The figure shows three views and two pictorial views of one solid part (mm, origin at its lowest corner). Answer the questions. Coordinates: 2 decimals unless noted, no trailing zeros. Loops run counter-clockwise (first coordinate to the right, second up) from the corner with the lowest first, then second, coordinate; pieces in that order, holes last. Notation, with made-up numbers: M 46.5,-7 L 104.5,-7 A22 ccw 104.5,25 Z; hole C -32.5,21 d9. An arc over 180 degrees is marked long. Return JSON: item names as keys, results as strings. Group by question number.
1. Section C-C (x = 32.25) is taken. Write down the section's boundary in (y, z).
2. Section D-D (z = 30) is taken. Write down the section's boundary in (x, y), then the cut area to 3 significant figures.
3. Given P1, Ø6, axis at x = 36.5, y = 23, coming from the -Z side; P2, Ø1, axis at x = 69.5, z = 93.5, coming from the +Y side; P3, Ø4, axis at y = 28.5, z = 33.5, coming from the -X side, each flat-ended and moving along its own axis, determine where each tip first touches the part or whether it passes through.
4. The mould has two halves that part along X. Classify the marked faces 1 and 2: pulls with the +X half, pulls with the -X half, needs draft (parallel to the pull), parting line crosses it, or undercut.
5. Section B-B (y = 32) is taken. Write down the section's boundary in (x, z), then the cut area to 3 significant figures.
6. Straight lines are drawn through the part: L1, parallel to Y at x = 89, z = 95; L2, parallel to X at y = 29, z = 33.5; L3, parallel to X at y = 19.5, z = 28. For each, find the intervals that lie inside material, in ascending order. Write a range as from..to.
7. Section A-A (z = 90) is taken. Write down the section's boundary in (x, y).
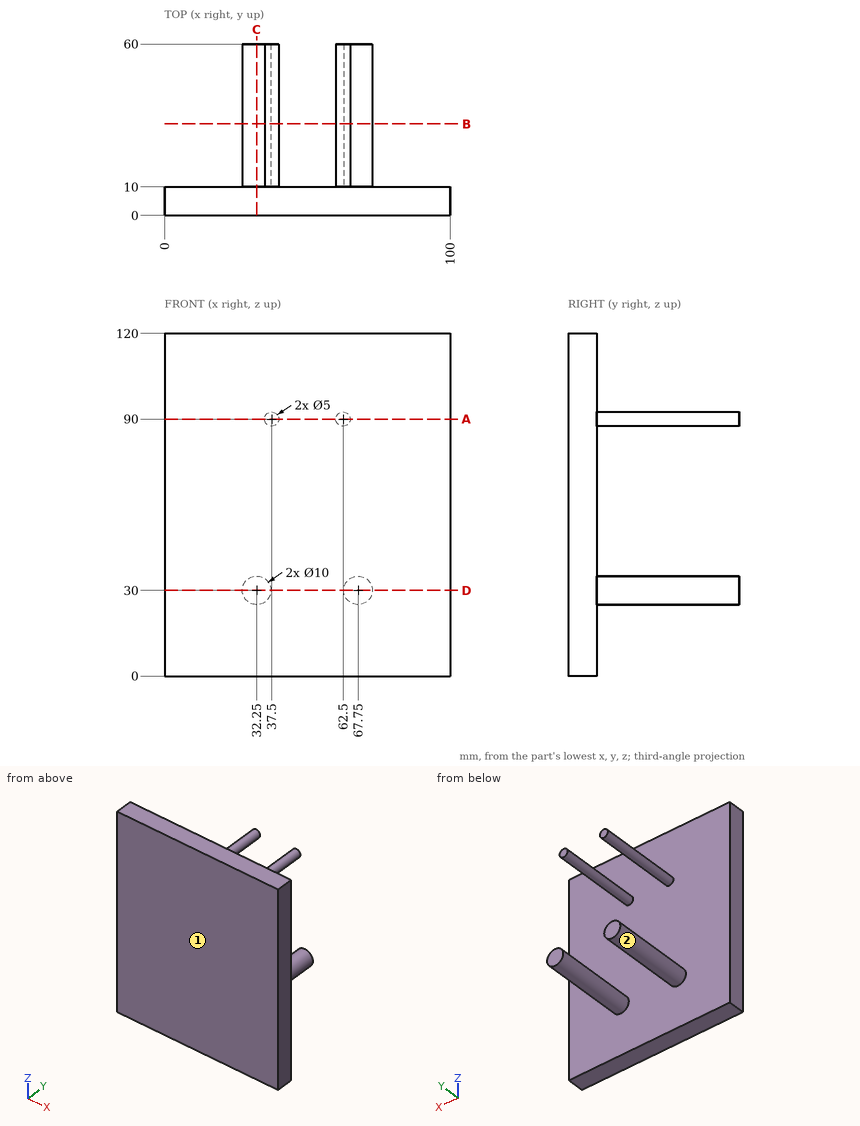
Worked out:
{
 "1": {"outline": "M 0,0 L 10,0 L 10,25 L 60,25 L 60,35 L 10,35 L 10,120 L 0,120 Z"},
 "2": {"outline": "M 0,0 L 100,0 L 100,10 L 72.75,10 L 72.75,60 L 62.75,60 L 62.75,10 L 37.25,10 L 37.25,60 L 27.25,60 L 27.25,10 L 0,10 Z", "area": "2,000 mm^2"},
 "3": {"P1": "z = 25.16", "P2": "y = 10", "P3": "x = 27.48"},
 "4": {"face 1": "needs draft", "face 2": "undercut"},
 "5": {"outline": "C 32.25,30 d10; C 37.5,90 d5; C 62.5,90 d5; C 67.75,30 d10", "area": "196 mm^2"},
 "6": {"L1": "0..10", "L2": "28.68..35.82, 64.18..71.32", "L3": "27.67..36.83, 63.17..72.33"},
 "7": {"outline": "M 0,0 L 100,0 L 100,10 L 65,10 L 65,60 L 60,60 L 60,10 L 40,10 L 40,60 L 35,60 L 35,10 L 0,10 Z"}
}
